Part model, mm, in its own coordinate system. Face numbers are marked on the shaded views. Give positions to 0.01 mm unless a question says otherwise; leave off trailing zeros. Order: outer loops, then holes, each group sorted by start corner. A loop starts at its lowest first (then second) coordinate and runs counter-clockwise, first axis right, second up. Notation, with made-up numbers: M 27.25,-1.5 L 62.25,-1.5 A22 cw 62.25,30.5 Z; hole C 18.5,12 d11. An arc over 180 degrees is marked long. Return JSON: item names as keys, results as strings.
from build123d import *

# Parameters (mm, degrees)
BOSS_EXTRUDE1_DEPTH = 228.6
SKETCH2_R           = 25.4
BOSS_EXTRUDE2_DEPTH = 12.7
SKETCH3_R           = 25.4
BOSS_EXTRUDE3_DEPTH = 12.7


with BuildPart() as part:
    # Sketch1 → Boss-Extrude1 (new body)
    with BuildSketch(Plane.XY):
        Polygon((-3.175, 5.499261314), (-6.35, 0), (-3.175, -5.499261314), (3.175, -5.499261314), (6.35, 0), (3.175, 5.499261314), align=None)
    extrude(amount=BOSS_EXTRUDE1_DEPTH)

    # Sketch2 → Boss-Extrude2 (add)
    with BuildSketch(Plane.XY.offset(85.725)):
        Circle(SKETCH2_R)
    extrude(amount=-BOSS_EXTRUDE2_DEPTH)

    # Sketch3 → Boss-Extrude3 (add)
    with BuildSketch(Plane.XY.offset(142.875)):
        Circle(SKETCH3_R)
    extrude(amount=BOSS_EXTRUDE3_DEPTH)


solid = part.part
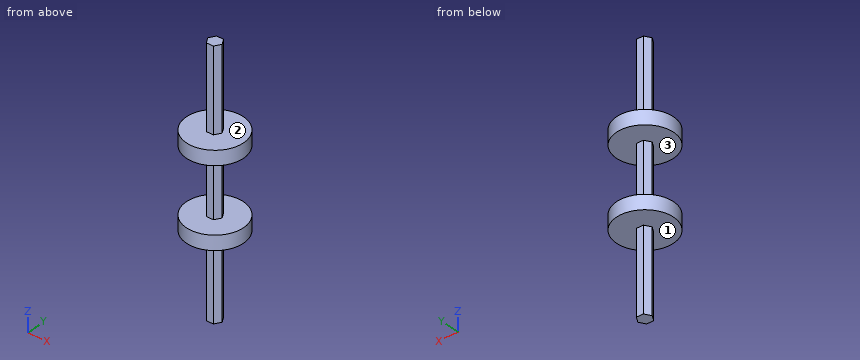
Q1. Band-saw the part on D-D (x = 0). Give the cut face in (y, z) (3 decimals).
Established:
{"outline": "M -25.4,73.025 L -5.499,73.025 L -5.499,0 L 5.499,0 L 5.499,73.025 L 25.4,73.025 L 25.4,85.725 L 5.499,85.725 L 5.499,142.875 L 25.4,142.875 L 25.4,155.575 L 5.499,155.575 L 5.499,228.6 L -5.499,228.6 L -5.499,155.575 L -25.4,155.575 L -25.4,142.875 L -5.499,142.875 L -5.499,85.725 L -25.4,85.725 Z"}
Q2. Band-saw the part on B-B (x = -14). Give the cut face in (y, z) (3 decimals).
Established:
{"outline": "M -21.193,73.025 L 21.193,73.025 L 21.193,85.725 L -21.193,85.725 Z; M -21.193,142.875 L 21.193,142.875 L 21.193,155.575 L -21.193,155.575 Z"}
Q3. Probe line 1 along Z through (x, y) = (-15, -9.5) (3 decimals); line 2 along Y through (x, z) = (-2.5, 69.5); line 3 along X through (y, z) = (0, 19.5). List the from-to ranges inside material, lowest first.
Established:
{"line 1": "z = 73.025 to 85.725, 142.875 to 155.575", "line 2": "y = -5.5 to 5.5", "line 3": "x = -6.35 to 6.35"}
Q4. Band-saw the part on A-A (y = 11). Give the cut face in (x, z) (3 decimals), then the cut area to 3 significant figures.
Established:
{"outline": "M -22.895,73.025 L 22.895,73.025 L 22.895,85.725 L -22.895,85.725 Z; M -22.895,142.875 L 22.895,142.875 L 22.895,155.575 L -22.895,155.575 Z", "area": "1,160 mm²"}
Q5. Pin check, flat tips, straight feed: pin 1 (3 mm diameter, centred on y = 8.5, z = 75.5, fed in from +X); pin 2 (1.9 mm diameter, centred on x = 1, z = 109.5, fed in from -Y); pin 3 (1.9 mm diameter, centred on x = -1.5, z = 101.5, fed in from +Y); pin 4 (12 mm diameter, centred on x = 18, z = 102.5, fed in from -Y). Stop position of each tip, or through.
Established:
{"pin 1": "stops at x = 24.42", "pin 2": "stops at y = -5.5", "pin 3": "stops at y = 5.5", "pin 4": "passes through"}
Q6. Two-plate mould, pull along Z, no slides. Class the marked faces 1, 2 and 3: +Z half, -Z half, draft (parallel to the pull), parting line (faces both ways), or undercut.
Established:
{"face 1": "-Z half", "face 2": "+Z half", "face 3": "undercut"}
Q7. Band-saw the part on C-C (z = 178). Give the cut face in (x, y) (3 decimals).
Established:
{"outline": "M -6.35,0 L -3.175,-5.499 L 3.175,-5.499 L 6.35,0 L 3.175,5.499 L -3.175,5.499 Z"}
